Work out the finished part from the listing and answer in its coordinate system (mm). A direction names the side the tool comes from. Round coordinates to 2 decimals unless told otherwise and drop trailing zeros. Loops run counter-clockwise (first coordinate to the right, second up) from the corner with the lowest first, then second, coordinate; pieces in that order, holes last. Notation, with made-up numbers: (28.5, 64) - (39.5, 64) arc R11 ccw to (39.5, 73) - close; hole circle Ø7 at (54, 68.5). An arc over 180 degrees is marked (long way). Answer as CSV lines item,"result". Start each with the question number.
Q1. Section C-C on x = 13.5 is taken. Write down the section's boundary in (y, z), then the cut area to 3 significant figures.
Q2. Section B-B on z = 0 is taken. Write down the section's boundary in (x, y), then the cut area to 3 significant figures.
Q3. Each of these flat-tipped pins is pushed along its axis until it touches: pin 1 Ø2 at (y, z) = (3, -10) entering from -X; pin 2 Ø6 at (x, z) = (32.5, -2.5) entering from -Y; pin 3 Ø4 at (x, y) = (42, 6) entering from -Z; pin 4 Ø4 at (x, z) = (13, 8) entering from +Y. Where does it stop, or does it pass through?
Q4. Section D-D on y = 13.25 is taken. Write down the section's boundary in (x, z), then the cut area to 3 significant figures.
Q5. For faces 4 (the face through (44, 0, -7)), 5 (the face through (29.13, -2.38, -10.74)), 6 (the face through (42, 0, 1.5)), 7 (the face through (20, 2, -8)), determine the directions among +Z, -Z, +X, -X, +Y, -Y from which every point of the face is accessible in a straight line to the end or side of a thin tool.
Q6. Section A-A on y = 0 is taken. Write down the section's boundary in (x, z), then the cut area to 4 significant figures.
Q7. Straight lines are drawn through the part: L1, parallel to X at y = -3.25, z = -8.25; L2, parallel to X at y = 11, z = -6; L3, parallel to Y at x = 25, z = -0.5. For each, find the intervals that lie inside material, in ascending order. Write a range as [from, to].
Q8. The mould has two halves that part along Z. Classify faces 1 (the face through (0, 0, 0)), 2 (the face through (42, 0, -1.5)), 3 (the face through (41.042, 13.856, -5.745)): +Z half, -Z half, draft (parallel to the pull), parting line (faces both ways), or undercut.
```python
from build123d import *

# Parameters (mm, degrees)
SKETCH2_W          = 3
SKETCH2_H          = 33.9969588
CUT_EXTRUDE1_DEPTH = 3.5


with BuildPart() as part:
    # Sketch1 → Revolve1 (revolve)
    with BuildSketch(Plane.XY):
        Polygon((0, 0), (0, 10), (17, 10), (17, 8), (20, 8), (20, 11), (38, 11), (38, 15), (44, 15), (44, 0), align=None)
    revolve(axis=Axis((0, 0, 0), (1, 0, 0)))

    # Sketch2 → Cut-Extrude1 (cut)
    with BuildSketch(Plane(origin=(44, 0, 0), x_dir=(0, 0, -1), z_dir=(1, 0, 0))):
        Rectangle(SKETCH2_W, SKETCH2_H)
    extrude(amount=-CUT_EXTRUDE1_DEPTH, mode=Mode.SUBTRACT)


solid = part.part
```
Findings:
1,outline,"circle Ø20 at (0, 0)"
1,area,"314 mm^2"
2,outline,"(0, -10) - (17, -10) - (17, -8) - (20, -8) - (20, -11) - (38, -11) - (38, -15) - (40.5, -15) - (40.5, 15) - (38, 15) - (38, 11) - (20, 11) - (20, 8) - (17, 8) - (17, 10) - (0, 10) - close"
2,area,"859 mm^2"
3,pin 1,"stops at x = 0"
3,pin 2,"stops at y = -11"
3,pin 3,"stops at z = -14.46"
3,pin 4,"stops at y = 8"
4,outline,"(38, -7.03) - (44, -7.03) - (44, -1.5) - (40.5, -1.5) - (40.5, 1.5) - (44, 1.5) - (44, 7.03) - (38, 7.03) - close"
4,area,"73.9 mm^2"
5,face 4,"+Z, -Z, +X, +Y, -Y"
5,face 5,"-X"
5,face 6,"+X, +Y, -Y"
5,face 7,"none"
6,outline,"(0, -10) - (17, -10) - (17, -8) - (20, -8) - (20, -11) - (38, -11) - (38, -15) - (44, -15) - (44, -1.5) - (40.5, -1.5) - (40.5, 1.5) - (44, 1.5) - (44, 15) - (38, 15) - (38, 11) - (20, 11) - (20, 8) - (17, 8) - (17, 10) - (0, 10) - close"
6,area,"953.5 mm^2"
7,L1,"x = [0, 17], [20, 44]"
7,L2,"x = [38, 44]"
7,L3,"y = [-10.99, 10.99]"
8,face 1,"draft"
8,face 2,"undercut"
8,face 3,"parting line"
